Autodesk Inventor part; units mm, degrees
ref_plane "YZ Plane" through (0, 0, 0) normal (1, 0, 0) x (0, 1, 0)
ref_plane "XZ Plane" through (0, 0, 0) normal (0, 1, 0) x (-1, 0, 0)
ref_plane "XY Plane" through (0, 0, 0) normal (0, 0, 1) x (1, 0, 0)
sketch "Sketch8" plane through (0, 0, 0) normal (0, 1, 0) x (-1, 0, 0)
  line L0 (45, -75) -> (45, 75)
  line L1 (45, 75) -> (-45, 75)
  line L2 (-45, 75) -> (-45, -75)
  line L3 (-45, -75) -> (45, -75)
  line L4 (-27.286, -57.286) -> (-27.286, -2.714)
  line L5 (27.286, -57.286) -> (-27.286, -57.286)
  line L6 (27.286, -2.714) -> (27.286, -57.286)
  line L7 (-27.286, -2.714) -> (27.286, -2.714)
  line L8 (27.286, 57.286) -> (27.286, 2.714)
  line L9 (27.286, 2.714) -> (-27.286, 2.714)
  line L10 (-27.286, 57.286) -> (27.286, 57.286)
  line L11 (-27.286, 2.714) -> (-27.286, 57.286)
  point P0 (0, 0)
extrude "Extrusion7" add sketch "Sketch8" against normal blind 10
sketch "Sketch2" plane through (0, 0, 0) normal (0, 1, 0) x (-1, 0, 0)
  line L0 (45, 75) -> (-45, 75)
  line L1 (-45, -75) -> (45, -75)
  line L2 (45, -75) -> (45, 75)
  line L3 (-45, 75) -> (-45, -75)
  line L4 (-25, -55) -> (25, -55)
  line L5 (25, -55) -> (25, -5)
  line L6 (25, -5) -> (-25, -5)
  line L7 (-25, -5) -> (-25, -55)
  line L8 (-25, 5) -> (25, 5)
  line L9 (25, 5) -> (25, 55)
  line L10 (25, 55) -> (-25, 55)
  line L11 (-25, 55) -> (-25, 5)
  line L12 (-27.286, 57.286) -> (27.286, 57.286)
  line L13 (27.286, 57.286) -> (27.286, 2.714)
  line L14 (27.286, 2.714) -> (-27.286, 2.714)
  line L15 (-27.286, 2.714) -> (-27.286, 57.286)
  line L16 (-27.286, -2.714) -> (27.286, -2.714)
  line L17 (27.286, -2.714) -> (27.286, -57.286)
  line L18 (27.286, -57.286) -> (-27.286, -57.286)
  line L19 (-27.286, -57.286) -> (-27.286, -2.714)
  point P0 (0, 0)
extrude "Extrusion8" add sketch "Sketch2" along normal blind 3 contours L2 L1 L3 L0 | L12 L13 L14 L15 | L16 L17 L18 L19
hole "Hole1" at (27.286, -5, 12.714) at (27.286, -5, 47.286) at (27.286, -5, -12.714) at (27.286, -5, -47.286) direction (1, 0, 0) diameter 5 depth 5 tip angle 118
hole "Hole2" at (-15.1837, -5, -57.286) at (17.1102, -5, -57.286) direction (0, 0, -1) diameter 5 depth 5 tip angle 118
hole "Hole3" at (-27.286, -5, 47.286) at (-27.286, -5, 12.714) at (-27.286, -5, -12.714) at (-27.286, -5, -47.286) direction (-1, 0, 0) diameter 5 depth 5 tip angle 118
hole "Hole5" at (17.1102, -5, 57.286) at (-15.1837, -5, 57.286) direction (0, 0, 1) diameter 5 depth 5 tip angle 118
hole "Hole6" at (-15.1837, -5, -2.714) at (17.1102, -5, -2.714) direction (0, 0, 1) diameter 5 end up to surface
properties part number "top_plate"
Here's how the part is built. I have some questions about the finished solid (model axes, mm). A direction names the side the tool comes from. Coordinates: 2 decimals unless noted, no trailing zeros. Order: outer loops, then holes, each group sorted by start corner. A loop starts at its lowest first (then second) coordinate and runs counter-clockwise, first axis right, second up.
1) Imagine slicing it at A-A on x = -6. List the corners of the cut face in (y, z) for me.
2) I need wall thicknesses on line 1 (Z direction, x = -28.4, y = -5); line 2 (Z direction, x = -8, y = -2); line 3 (X direction, y = -5, z = -58.45). Which ranges of each line are inside material? Lowest first, please.
3) Imagine slicing it at B-B on z = -26. List the corners of the cut face in (x, y) for me, and give its area (3 significant figures).
4) We'd pull the mould along Y, two halves only. Please class faces 1 (the face through (-29.821, -5.11, 49.784)), 2 (the face through (27.286, -5, 30)), 3 (the face through (1, -10, 1)): +Y half, -Y half, draft (parallel to the pull), parting line (faces both ways), or undercut.
5) Imagine slicing it at C-C on x = -29. List the corners of the cut face in (y, z) for me.
6) Which directions (+Z, -Z, +X, -X, +Y, -Y) give clear straight access to the entire face, cutting with the end or side of a thin tool? Please do faces 4 (the face through (-27.286, -5, 30)), 5 (the face through (-25, 1, 30)), 6 (the face through (29.821, -5.11, -49.784)).
Response values:
1. outline: (-10, -75) - (3, -75) - (3, -55) - (0, -55) - (0, -57.29) - (-10, -57.29) - close; (-10, -2.71) - (0, -2.71) - (0, -5) - (3, -5) - (3, 5) - (0, 5) - (0, 2.71) - (-10, 2.71) - close; (-10, 57.29) - (0, 57.29) - (0, 55) - (3, 55) - (3, 75) - (-10, 75) - close
2. line 1: z = -75 to -49.79, -44.79 to -15.21, -10.21 to 10.21, 15.21 to 44.79, 49.79 to 75
2. line 2: z = -75 to -57.29, -2.71 to 2.71, 57.29 to 75
2. line 3: x = -45 to -17.68, -12.68 to 14.61, 19.61 to 45
3. outline: (-45, -10) - (-27.29, -10) - (-27.29, 0) - (-25, 0) - (-25, 3) - (-45, 3) - close; (25, 0) - (27.29, 0) - (27.29, -10) - (45, -10) - (45, 3) - (25, 3) - close
3. area: 474 mm2
4. face 1: undercut
4. face 2: draft
4. face 3: -Y half
5. outline: (-10, -75) - (3, -75) - (3, 75) - (-10, 75) - close; hole circle Ø5 at (-5, -47.29); hole circle Ø5 at (-5, -12.71); hole circle Ø5 at (-5, 12.71); hole circle Ø5 at (-5, 47.29)
6. face 4: -Y
6. face 5: +Y, -Y
6. face 6: none
